For this review, take the finished solid that the model builds, in its own axes (mm). Give positions to 0.01 mm unless a question says otherwise; leave off trailing zeros. Order: outer loops, then holes, each group sorted by start corner. A loop starts at its lowest first (then second) coordinate and runs counter-clockwise, first axis right, second up. Notation, with made-up numbers: M 60,81 L 110,81 A25 cw 110,102 Z; hole C 14.5,82 d8. An arc over 180 degrees is marked long. Use CSV: the item, a comma, the result in double quotes. Start each with the question number.
(1) Consider section C-C (x = -59). Write out the cut boundary in (y, z), and give its area (3 significant figures).
(2) Consider section D-D (z = 81). Write out the cut boundary in (x, y), and give its area (3 significant figures).
(3) Clearance check with flat-ended pins moving along their axes: P1, Ø2.5, axis at x = -137.5, y = -3, coming from the +Z side; P2, Ø4.5, axis at y = -3.5, z = 90, coming from the -X side. State where each tip first meets the part, or that it passes through.
(4) Consider section B-B (y = -4.5). Write out the cut boundary in (x, z).
(5) Wall thickness on L1, parallel to X at y = -4.75, z = 75; L2, parallel to X at y = -8.5, z = 54.5; L3, parallel to X at y = -1, z = 88.5: over which ranges is each line inside the solid? List them lowest first. Write a range as from..to.
(6) Consider section A-A (z = 57.5). Write out the cut boundary in (x, y).
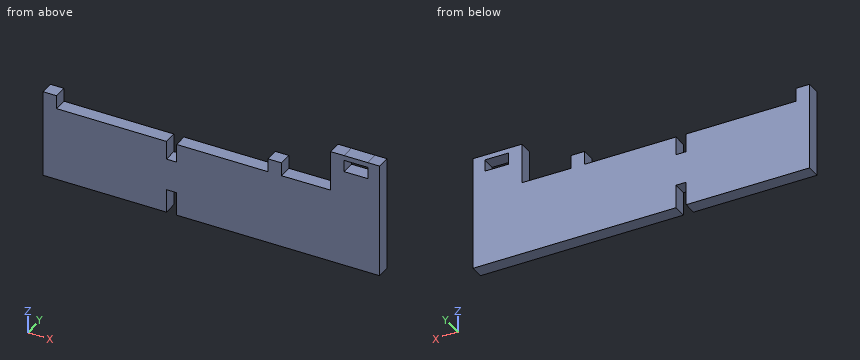
```python
from build123d import *

# Parameters (mm, degrees)
F1_DEPTH = 10.16


with BuildPart() as f1:
    # F0 (on Front) → F1 (new body)
    with BuildSketch(Plane.XZ):
        Polygon((-134.797797, 11.368327), (12.51955, 11.368327), (17.712758, 11.368327), (17.712758, 98.023848), (8.808348, 97.969344), (8.831047, 94.261023), (8.831047, 85.363727), (-8.979842, 85.254705), (-9.034301, 94.151668), (-9.057669, 97.969344), (-19.210024, 97.9072), (-19.210024, 67.486234), (-56.051124, 67.260727), (-56.051124, 77.432118), (-66.21471, 77.432118), (-66.21471, 67.260727), (-134.797797, 67.260727), (-134.797797, 53.284746), (-142.41989, 53.284746), (-142.41989, 67.260727), (-224.99001, 67.260727), (-224.99001, 77.432118), (-235.15287, 77.432118), (-235.15287, 11.368327), (-142.41989, 11.368327), (-142.41989, 29.144347), (-134.797797, 29.144347), align=None)
        Polygon((8.831047, 94.261023), (8.808348, 97.969344), (-9.057669, 97.969344), (-9.034301, 94.151668), align=None)
    extrude(amount=F1_DEPTH)


solid = f1.part
```
Check result:
1,outline,"M -10.16,11.37 L 0,11.37 L 0,77.43 L -10.16,77.43 Z"
1,area,"671 mm^2"
2,outline,"M -19.21,-10.16 L 17.71,-10.16 L 17.71,0 L -19.21,0 Z"
2,area,"375 mm^2"
3,P1,"stops at z = 53.28"
3,P2,"stops at x = -19.21"
4,outline,"M -235.15,11.37 L -142.42,11.37 L -142.42,29.14 L -134.8,29.14 L -134.8,11.37 L 17.71,11.37 L 17.71,98.02 L 8.81,97.97 L -9.06,97.97 L -19.21,97.91 L -19.21,67.49 L -56.05,67.26 L -56.05,77.43 L -66.21,77.43 L -66.21,67.26 L -134.8,67.26 L -134.8,53.28 L -142.42,53.28 L -142.42,67.26 L -224.99,67.26 L -224.99,77.43 L -235.15,77.43 Z; hole M -9.03,94.15 L -8.98,85.25 L 8.83,85.36 L 8.83,94.26 Z"
5,L1,"x = -235.15..-224.99, -66.21..-56.05, -19.21..17.71"
5,L2,"x = -235.15..-142.42, -134.8..17.71"
5,L3,"x = -19.21..-9, 8.83..17.71"
6,outline,"M -235.15,-10.16 L -142.42,-10.16 L -142.42,0 L -235.15,0 Z; M -134.8,-10.16 L 17.71,-10.16 L 17.71,0 L -134.8,0 Z"
